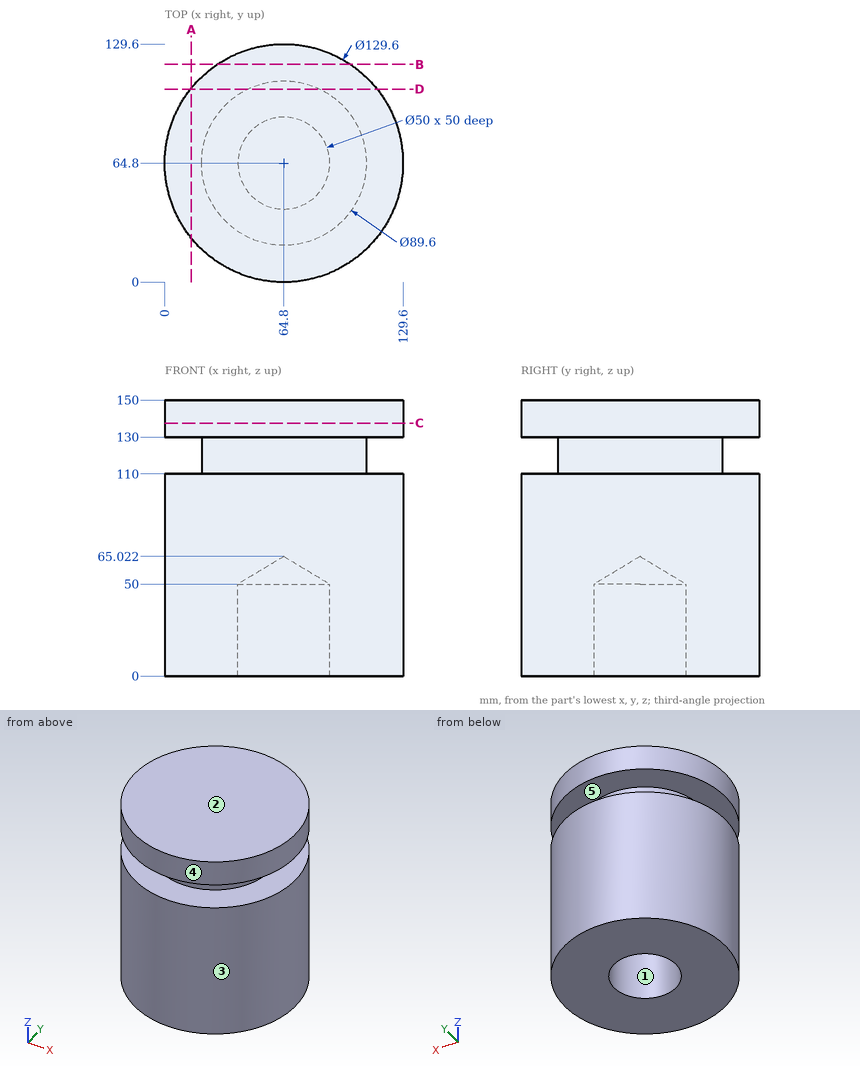
Input: dimensioned drawing with shaded views. Units: mm. Origin: part minimum x, y, z. A direction names the side the tool comes from. Round coordinates to 2 decimals unless told otherwise and drop trailing zeros. Loops run counter-clockwise (first coordinate to the right, second up) from the corner with the lowest first, then second, coordinate; pieces in that order, holes last. Notation, with made-up numbers: M 87.25,-19 L 112.25,-19 A13 ccw 112.25,-12 Z; hole C 38,63 d1. An arc over 180 degrees is marked long. Return JSON: item names as keys, results as strings. Group by question number.
1. Material intervals for line 1 along Z through (x, y) = (62.5, 14); line 2 along X through (y, z) = (64, 31) (1 decimal), sorted ascending. Write a range as from..to.
2. Pin query (flat end, axial travel): pin 1 (2 mm diameter, centred on x = 77.5, z = 95.5, fed in from -Y) (1 decimal); pin 2 (3 mm diameter, centred on x = 69.5, z = 89.5, fed in from -Y); pin 3 (3 mm diameter, centred on y = 26.5, z = 127, fed in from +X). Return the tip coordinate at first contact, or that it passes through.
3. Section query D-D on y = 105. Output: boundary loops of the cut face in (x, z), and give its area (3 significant figures).
4. Section query B-B on y = 118.5. Output: boundary loops of the cut face in (x, z).
5. Reachability of the marked faces 4 and 5 from +Z, -Z, +X, -X, +Y, -Y: full face, straight path, thin tool, end or side. Return the list, or none.
6. Mould query, pull axis Y, two halves, no side actions, for the marked faces 1, 2 and 3. Classes: released by +Y, released by -Y, zero draft, split by the parting line, or undercut.
7. Section query C-C on z = 137.5. Output: boundary loops of the cut face in (x, y).
8. Section query A-A on x = 14.5. Output: boundary loops of the cut face in (y, z), and give its area (3 significant figures).
Checks:
{
 "1": {"line 1": "z = 0..110, 130..150", "line 2": "x = 0..39.8, 89.8..129.6"},
 "2": {"pin 1": "stops at y = 1.1", "pin 2": "stops at y = 0.08", "pin 3": "stops at x = 90.35"},
 "3": {"outline": "M 13.98,0 L 115.62,0 L 115.62,110 L 84.57,110 L 84.57,130 L 115.62,130 L 115.62,150 L 13.98,150 L 13.98,130 L 45.03,130 L 45.03,110 L 13.98,110 Z", "area": "14,000 mm²"},
 "4": {"outline": "M 28.53,0 L 101.07,0 L 101.07,110 L 28.53,110 Z; M 28.53,130 L 101.07,130 L 101.07,150 L 28.53,150 Z"},
 "5": {"face 4": "+Z, -Z", "face 5": "none"},
 "6": {"face 1": "undercut", "face 2": "zero draft", "face 3": "split by the parting line"},
 "7": {"outline": "C 64.8,64.8 d129.6"},
 "8": {"outline": "M 23.95,0 L 105.65,0 L 105.65,110 L 23.95,110 Z; M 23.95,130 L 105.65,130 L 105.65,150 L 23.95,150 Z", "area": "10,600 mm²"}
}
